```python
from build123d import *

# Parameters (mm, degrees)
ESQUISSE1_W              = 39.5
ESQUISSE1_H              = 32.5
BOSS_EXTRU_1_DEPTH       = 14
ESQUISSE2_W              = 37.4
ESQUISSE2_H              = 30.6
ENL_V_MAT_EXTRU_1_DEPTH  = 13
ESQUISSE3_W              = 4
ESQUISSE3_H              = 28.5
ENL_V_MAT_EXTRU_2_DEPTH  = 5
ESQUISSE4_W              = 12.5
ESQUISSE4_H              = 26.5
ENL_V_MAT_EXTRU_3_DEPTH  = 5
ESQUISSE6_W              = 14.8
ESQUISSE6_H              = 14.8
ENL_V_MAT_EXTRU_5_DEPTH  = 53.777836257
ESQUISSE7_W              = 9.75
ESQUISSE7_H              = 23.1
ENL_V_MAT_EXTRU_6_DEPTH  = 53.777836257
ESQUISSE8_W              = 4
ESQUISSE8_H              = 22.8
BOSS_EXTRU_3_DEPTH       = 1
ESQUISSE8_2_W            = 4
ESQUISSE8_2_H            = 22.8
ENL_V_MAT_EXTRU_7_DEPTH  = 1
ESQUISSE9_W              = 3
ESQUISSE9_H              = 22.8
ENL_V_MAT_EXTRU_9_DEPTH  = 1.2
BOSS_EXTRU_6_DEPTH       = 2
BOSS_EXTRU_7_DEPTH       = 2
ESQUISSE14_W             = 40
ESQUISSE14_H             = 9.401923789
ENL_V_MAT_EXTRU_10_DEPTH = 54.033008589
ESQUISSE15_W             = 3.5
ESQUISSE15_H             = 4
ENL_V_MAT_EXTRU_11_DEPTH = 54.033008589
CHANFREIN1_SIZE          = 0.352653961
CHANFREIN1_SIZE_2        = 2


with BuildPart() as part:
    # Esquisse1 → Boss.-Extru.1 (new body)
    with BuildSketch(Plane.XY):
        with Locations((19.75, 16.25)):
            Rectangle(ESQUISSE1_W, ESQUISSE1_H)
    extrude(amount=BOSS_EXTRU_1_DEPTH)

    # Esquisse2 → Enlèv. mat.-Extru.1 (cut)
    with BuildSketch(Plane.XY.offset(14)):
        with Locations((19.65, 16.15)):
            Rectangle(ESQUISSE2_W, ESQUISSE2_H)
    extrude(amount=-ENL_V_MAT_EXTRU_1_DEPTH, mode=Mode.SUBTRACT)

    # Esquisse3 → Enlèv. mat.-Extru.2 (cut)
    with BuildSketch(Plane(origin=(39.5, 0, 0), x_dir=(0, 0, -1), z_dir=(1, 0, 0))):
        with Locations((-12, 16.25)):
            Rectangle(ESQUISSE3_W, ESQUISSE3_H)
    extrude(amount=-ENL_V_MAT_EXTRU_2_DEPTH, mode=Mode.SUBTRACT)

    # Esquisse4 → Enlèv. mat.-Extru.3 (cut)
    with BuildSketch(Plane.ZY):
        with Locations((7.75, 16.25)):
            Rectangle(ESQUISSE4_W, ESQUISSE4_H)
    extrude(amount=-ENL_V_MAT_EXTRU_3_DEPTH, mode=Mode.SUBTRACT)

    # Esquisse6 → Enlèv. mat.-Extru.5 (cut, through all)
    with BuildSketch(Plane.XY.offset(1)):
        with Locations((27.1, 9.4)):
            Rectangle(ESQUISSE6_W, ESQUISSE6_H)
    extrude(amount=-ENL_V_MAT_EXTRU_5_DEPTH, mode=Mode.SUBTRACT)

    # Esquisse7 → Enlèv. mat.-Extru.6 (cut, through all)
    with BuildSketch(Plane.XY.offset(1)):
        with Locations((7.625, 16.25)):
            Rectangle(ESQUISSE7_W, ESQUISSE7_H)
    extrude(amount=-ENL_V_MAT_EXTRU_6_DEPTH, mode=Mode.SUBTRACT)

    # Esquisse8 → Boss.-Extru.3 (add)
    with BuildSketch(Plane(origin=(0, 0, 0), x_dir=(-1, 0, 0), z_dir=(0, 0, -1))):
        with Locations((-37.5, 16.2)):
            Rectangle(ESQUISSE8_W, ESQUISSE8_H)
    extrude(amount=-BOSS_EXTRU_3_DEPTH)

    # Esquisse8<2> → Enlèv. mat.-Extru.7 (cut)
    with BuildSketch(Plane(origin=(0, 0, 0), x_dir=(-1, 0, 0), z_dir=(0, 0, -1))):
        with Locations((-37.5, 16.2)):
            Rectangle(ESQUISSE8_2_W, ESQUISSE8_2_H)
    extrude(amount=-ENL_V_MAT_EXTRU_7_DEPTH, mode=Mode.SUBTRACT)

    # Esquisse9 → Enlèv. mat.-Extru.9 (cut)
    with BuildSketch(Plane(origin=(39.5, 0, 0), x_dir=(0, 0, -1), z_dir=(1, 0, 0))):
        with Locations((-2.5, 16.2)):
            Rectangle(ESQUISSE9_W, ESQUISSE9_H)
    extrude(amount=-ENL_V_MAT_EXTRU_9_DEPTH, mode=Mode.SUBTRACT)

    # Esquisse12 → Boss.-Extru.6 (add)
    with BuildSketch(Plane(origin=(0, 32.5, 0), x_dir=(1, 0, 0), z_dir=(0, 1, 0))):
        Polygon((0, 0), (-0.001437079, 12), (39.5, 10), (39.5, 0), align=None)
    extrude(amount=-BOSS_EXTRU_6_DEPTH)

    # Esquisse13 → Boss.-Extru.7 (add)
    with BuildSketch(Plane.XZ):
        Polygon((39.5, 0), (39.5, -9.999999903), (0, -12), (0, 0), align=None)
    extrude(amount=-BOSS_EXTRU_7_DEPTH)

    # Esquisse14 → Enlèv. mat.-Extru.10 (cut, through all)
    with BuildSketch(Plane(origin=(0, 0, 0), x_dir=(-1, 0, 0), z_dir=(0, -1, 0))):
        with Locations((-19.5, 8.165063509)):
            Rectangle(ESQUISSE14_W, ESQUISSE14_H)
    extrude(amount=-ENL_V_MAT_EXTRU_10_DEPTH, mode=Mode.SUBTRACT)

    # Esquisse15 → Enlèv. mat.-Extru.11 (cut, through all)
    with BuildSketch(Plane(origin=(0, 0, 0), x_dir=(-1, 0, 0), z_dir=(0, -1, 0))):
        with Locations((-16.75, 2.218139361)):
            Rectangle(ESQUISSE15_W, ESQUISSE15_H)
    extrude(amount=-ENL_V_MAT_EXTRU_11_DEPTH, mode=Mode.SUBTRACT)

    # Chanfrein1
    # the kernel refuses this chamfer: 2, 0.352653961 mm, written as the material it takes off along each edge
    with BuildSketch(Plane(origin=(-5.197077593, 0, -3.464101615), x_dir=(0, -0.21013876076743054, 0.9776715712462588), z_dir=(1, 0, 0))) as chanfrein1_piece_1:
        Polygon((CHANFREIN1_SIZE * 0.977671572402, -CHANFREIN1_SIZE * 0.210138761016), (-CHANFREIN1_SIZE_2 * 0.210138760767, -CHANFREIN1_SIZE_2 * 0.977671571246), (0, 0), align=None)
    extrude(amount=25.394155186, mode=Mode.SUBTRACT)
    with BuildSketch(Plane(origin=(13.302922407, 0, -3.464101615), x_dir=(0, -0.2101387607674303, 0.9776715712462589), z_dir=(1, 0, 0))) as chanfrein1_piece_2:
        Polygon((CHANFREIN1_SIZE * 0.977671572402, -CHANFREIN1_SIZE * 0.210138761016), (-CHANFREIN1_SIZE_2 * 0.210138760767, -CHANFREIN1_SIZE_2 * 0.977671571246), (0, 0), align=None)
    extrude(amount=31.394155186, mode=Mode.SUBTRACT)
    with BuildSketch(Plane(origin=(-5.197492442, 32.5, -3.464101615), x_dir=(0, 0.21013876076742352, 0.9776715712462605), z_dir=(1, 0, 0))) as chanfrein1_piece_3:
        Polygon((CHANFREIN1_SIZE * 0.977671572402, CHANFREIN1_SIZE * 0.210138761016), (-CHANFREIN1_SIZE_2 * 0.210138760767, CHANFREIN1_SIZE_2 * 0.977671571246), (0, 0), align=None)
    extrude(amount=25.394570035, mode=Mode.SUBTRACT)
    with BuildSketch(Plane(origin=(13.302922407, 32.5, -3.464101615), x_dir=(0, 0.21013876076742327, 0.9776715712462605), z_dir=(1, 0, 0))) as chanfrein1_piece_4:
        Polygon((CHANFREIN1_SIZE * 0.977671572402, CHANFREIN1_SIZE * 0.210138761016), (-CHANFREIN1_SIZE_2 * 0.210138760767, CHANFREIN1_SIZE_2 * 0.977671571246), (0, 0), align=None)
    extrude(amount=31.394155186, mode=Mode.SUBTRACT)


solid = part.part
```
Check sheet for the modelled part. Datum: model origin and axes. Units: mm. A direction names the side the tool comes from. Give positions to 0.01 mm unless a question says otherwise; leave off trailing zeros. Order: outer loops, then holes, each group sorted by start corner. A loop starts at its lowest first (then second) coordinate and runs counter-clockwise, first axis right, second up. Notation, with made-up numbers: (-15, 29.5) -> (19, 29.5) arc R21 ccw to (19, 63.5) -> close; hole circle Ø10 at (-28.5, -22.5). An arc over 180 degrees is marked (long way). Use CSV: the item, a comma, the result in double quotes. Start each with the question number.
1) Mould release check, pull along X, two halves, no side actions. Record for faces 1 (the face through (35.5, 16, 0.5)), 2 (the face through (20, 30.5, -2)), 3 (the face through (19, 20, 1)): released by +X, released by -X, zero draft, split by the parting line, or undercut.
2) Sectioned sample at D-D, the plane y = 27. Record the boundary of the cut face in (x, z), plus the area to 3 significant figures.
3) Material ranges on line 1 (X direction, y = 12, z = 0.75); line 2 (Y direction, x = 7.5, z = 4.75); line 3 (X direction, y = 30.5, z = 3.25), recorded low to high. Write a range as from..to.
4) Set-up check for faces 4 (the face through (0.5, 29.5, 7.7)), 5 (the face through (16, 20, 0)), 6 (the face through (18.5, 31, -2)): record each of +Z, -Z, +X, -X, +Y, -Y from which the full face is reachable in a straight line by a thin tool's end or side.
5) Sectioned sample at A-A, the plane x = 7. Record the boundary of the cut face in (y, z).
6) Sectioned sample at B-B, the plane y = 15.5. Record the boundary of the cut face in (x, z), plus the area to 3 significant figures.
7) Go/stop test with flat-tipped pins: P1, Ø0.5, axis at y = 21, z = 0.5, coming from the +X side; P2, Ø6, axis at x = 14.5, y = 23, coming from the -Z side; P3, Ø1.5, axis at y = 4.5, z = 3, coming from the -X side; P4, Ø5, axis at y = 26, z = 3.5, coming from the +X side. Record where each tip stops, or that it passes through.
8) Sectioned sample at C-C, the plane z = 13. Record the boundary of the cut face in (x, y).
Recorded:
1,face 1,"released by +X"
1,face 2,"zero draft"
1,face 3,"undercut"
2,outline,"(0, 0) -> (2.75, 0) -> (2.75, 1) -> (0.95, 1) -> (0.95, 1.5) -> (0, 1.5) -> close; (12.5, 0) -> (35.5, 0) -> (35.5, 1) -> (12.5, 1) -> close; (38.35, 4) -> (39.5, 4) -> (39.5, 10) -> (38.35, 10) -> close"
2,area,"33.1 mm2"
3,line 1,"0..2.75, 12.5..19.7, 34.5..35.5"
3,line 2,"0..0.85, 31.45..32.5"
3,line 3,"0..0.95, 38.35..39.5"
4,face 4,"+Z, -X"
4,face 5,"-Z, +X, -X"
4,face 6,"-Z, +Y, -Y"
5,outline,"(0, -3.11) -> (2, -3.46) -> (2, 0) -> (4.7, 0) -> (4.7, 1) -> (0.85, 1) -> (0.85, 14) -> (0, 14) -> close; (27.8, 0) -> (30.5, 0) -> (30.5, -3.46) -> (32.5, -3.11) -> (32.5, 14) -> (31.45, 14) -> (31.45, 1) -> (27.8, 1) -> close"
6,outline,"(0, 0) -> (2.75, 0) -> (2.75, 1) -> (0.95, 1) -> (0.95, 1.5) -> (0, 1.5) -> close; (12.5, 0) -> (19.7, 0) -> (19.7, 1) -> (12.5, 1) -> close; (34.5, 0) -> (35.5, 0) -> (35.5, 1) -> (34.5, 1) -> close; (38.35, 4) -> (39.5, 4) -> (39.5, 10) -> (38.35, 10) -> close"
6,area,"18.3 mm2"
7,P1,"x = 35.5"
7,P2,"z = 0"
7,P3,"x = 38.35"
7,P4,"x = 39.5"
8,outline,"(0, 0) -> (39.5, 0) -> (39.5, 2) -> (38.35, 2) -> (38.35, 0.85) -> (0.95, 0.85) -> (0.95, 3) -> (0, 3) -> close; (0, 29.5) -> (0.95, 29.5) -> (0.95, 31.45) -> (38.35, 31.45) -> (38.35, 30.5) -> (39.5, 30.5) -> (39.5, 32.5) -> (0, 32.5) -> close"
